Can you work these out from the model? Positions are in its coordinate system, mm. A direction names the side the tool comes from. Coordinates: 2 decimals unless noted, no trailing zeros. Loops run counter-clockwise (first coordinate to the right, second up) from the corner with the lowest first, then second, coordinate; pieces in that order, holes last.
```python
from build123d import *

# Parameters (mm, degrees)
F4_DEPTH = 100.001
F5_SIZE  = 1


with BuildPart() as f1:
    # F0 (on Right) → F1 (revolve)
    with BuildSketch(Plane.YZ):
        Polygon((-142.5, 42.5), (-142.5, 0), (-42.5, 0), (-42.5, 42.5), (-67.5, 42.5), (-67.5, 51.5), (-103.5, 51.5), (-103.5, 42.5), (-131.5, 42.5), (-131.5, 40.75), (-134.65, 40.75), (-134.65, 42.5), align=None)
    revolve(axis=Axis((0, -92.5, 0), (0, -1, 0)))

    # F3 (on face) → F4 (cut, through all)
    with BuildSketch(Plane.XZ.offset(142.5)):
        with BuildLine():
            Line((-4, 35.5529068457), (-4, 32.2529068457))
            ThreePointArc((-4, 32.2529068457), (0, -32.5), (4, 32.2529068457))
            Line((4, 32.2529068457), (4, 35.5529068457))
            Line((4, 35.5529068457), (-4, 35.5529068457))
        make_face()
    extrude(amount=-F4_DEPTH, mode=Mode.SUBTRACT)

    # F5
    f5_edges = [f1.edges().sort_by_distance(p)[0] for p in [
        (0, -142.5, -42.5),
        (0, -42.5, -32.5),
    ]]
    chamfer(f5_edges, length=F5_SIZE)


solid = f1.part
```
(1) I'm going to push flat-ended pins straight in: pin 1 (12 mm diameter, centred on x = 15, z = 20, fed in from -Y); pin 2 (5 mm diameter, centred on x = -27.5, y = -105.5, fed in from -Z); pin 3 (1.5 mm diameter, centred on x = -5, y = -119.5, fed in from -Z); pin 4 (8 mm diameter, centred on x = 1.5, y = -57, fed in from -Z). Where does each tip first touch, or does it pass through?
Check values:
pin 1: passes through
pin 2: stops at z = -44.46
pin 3: stops at z = -42.29
pin 4: stops at z = -42.5
(2) If I drill on probe 1 along Z at (x, y) = (0, -72); probe 2 along X at (y, z) = (-104.5, 0); probe 3 along Z at (x, y) = (0, -119.5), over which ranges is the centre line in solid material (lowest first)?
Check values:
probe 1: z = -51.5 to -32.5, 35.55 to 51.5
probe 2: x = -42.5 to -32.5, 32.5 to 42.5
probe 3: z = -42.5 to -32.5, 35.55 to 42.5
(3) If we mould it in two halves opening along X, with no side actions, what happens to faces 1 (the cylindrical face through (25.861, -138.123, -33.727)), 2 (the flat face through (41, -134.65, -3)), 3 (the flat face through (4, -93, 34))? For each: released by +X, released by -X, zero draft, split by the parting line, or undercut.
Check values:
face 1: split by the parting line
face 2: zero draft
face 3: undercut
(4) I want a section at B-B on x = 0. Write out the boundary of the cut face in (y, z).
Check values:
outline: (-142.5, -41.5) - (-141.5, -42.5) - (-134.65, -42.5) - (-134.65, -40.75) - (-131.5, -40.75) - (-131.5, -42.5) - (-103.5, -42.5) - (-103.5, -51.5) - (-67.5, -51.5) - (-67.5, -42.5) - (-42.5, -42.5) - (-42.5, -33.5) - (-43.5, -32.5) - (-142.5, -32.5) - close; (-142.5, 35.55) - (-42.5, 35.55) - (-42.5, 42.5) - (-67.5, 42.5) - (-67.5, 51.5) - (-103.5, 51.5) - (-103.5, 42.5) - (-131.5, 42.5) - (-131.5, 40.75) - (-134.65, 40.75) - (-134.65, 42.5) - (-141.5, 42.5) - (-142.5, 41.5) - close
(5) I want a section at D-D on y = -50.5. Write out the boundary of the cut face in (x, z), then the cut area to 3 significant figures.
Check values:
outline: circle Ø85 at (0, 0); hole (-4, 32.25) arc R32.5 ccw (long way) to (4, 32.25) - (4, 35.55) - (-4, 35.55) - close
area: 2,330 mm2
(6) Which directions (+Z, -Z, +X, -X, +Y, -Y) give clear straight access to the entire face, cutting with the end or side of a thin tool? Please do faces 4 (the flat face through (41, -131.5, 3)), 5 (the flat face through (-42.2, -67.5, -7.4)), 6 (the flat face through (0, -93, 35.553)).
Check values:
face 4: none
face 5: +Y
face 6: +Y, -Y
(7) I want a section at C-C on y = -73.5. Write out the boundary of the cut face in (x, z).
Check values:
outline: circle Ø103 at (0, 0); hole (-4, 32.25) arc R32.5 ccw (long way) to (4, 32.25) - (4, 35.55) - (-4, 35.55) - close
(8) I want a section at A-A on z = 0. Write out the boundary of the cut face in (x, y).
Check values:
outline: (-51.5, -103.5) - (-42.5, -103.5) - (-42.5, -131.5) - (-40.75, -131.5) - (-40.75, -134.65) - (-42.5, -134.65) - (-42.5, -141.5) - (-41.5, -142.5) - (-32.5, -142.5) - (-32.5, -43.5) - (-33.5, -42.5) - (-42.5, -42.5) - (-42.5, -67.5) - (-51.5, -67.5) - close; (32.5, -142.5) - (41.5, -142.5) - (42.5, -141.5) - (42.5, -134.65) - (40.75, -134.65) - (40.75, -131.5) - (42.5, -131.5) - (42.5, -103.5) - (51.5, -103.5) - (51.5, -67.5) - (42.5, -67.5) - (42.5, -42.5) - (33.5, -42.5) - (32.5, -43.5) - close
